Design review of the part built by this model. Coordinates are the model's own, in mm. Face numbers are marked on the shaded views. A direction names the side the tool comes from. Round coordinates to 2 decimals unless told otherwise and drop trailing zeros. Loops run counter-clockwise (first coordinate to the right, second up) from the corner with the lowest first, then second, coordinate; pieces in that order, holes last. Notation, with made-up numbers: (-13, 84.25) - (2, 84.25) arc R13 ccw to (2, 96.25) - close; hole circle Ø6 at (77, 14.5). An arc over 180 degrees is marked (long way). Use one line per item in the form item = value. Start each with the question number.
(1) Machinability: for the marked faces 1 and 2, which of the approach directions +Z, -Z, +X, -X, +Y, -Y give a long, thin tool a straight path to every point of the face, cutting with its end or side? Answer none if there is none.
(2) We need section D-D, the plane y = -17. Write out the cut boundary in (x, z).
(3) Wall thickness on probe 1 along Z at (x, y) = (-7, -2); probe 2 along Z at (x, y) = (-7.5, -3.45); probe 3 along Y at (x, z) = (-6, 7): over which ranges is each line inside the solid? List them lowest first. Write a range as [from, to].
(4) We need section A-A, the plane x = -15. Write out the cut boundary in (y, z).
(5) For pin 1 (1.9 mm diameter, centred on x = -7.5, z = 12.99, fed in from -Y); pin 2 (3 mm diameter, centred on x = -10.5, z = 15, fed in from -Y); pin 3 (4 mm diameter, centred on x = -1, y = -33.5, fed in from +Z); pin 4 (12 mm diameter, centred on x = -8.5, y = -10.5, fed in from +Z), all flat-tipped, find the tip position at first contact; note any pin that passes through.
(6) We need section C-C, the plane z = -4. Write out the cut boundary in (x, y), then the cut area to 3 significant figures.
(7) We need section B-B, the plane x = 7.5. Write out the cut boundary in (y, z), then the cut area to 3 significant figures.
from build123d import *

# Parameters (mm, degrees)
F0_R     = 21
F0_R_2   = 2
F0_R_3   = 5
F1_DEPTH = 6
F2_DEPTH = 38
F3_D     = 3.2


with BuildPart() as f1:
    # F0 (on Front) → F1 (new body)
    with BuildSketch(Plane.XZ):
        Circle(F0_R)
        with Locations((-7.5, -12.9903810568)):
            Circle(F0_R_2, mode=Mode.SUBTRACT)
        with Locations((7.5, -12.9903810568)):
            Circle(F0_R_2, mode=Mode.SUBTRACT)
        with Locations((-15, 0)):
            Circle(F0_R_2, mode=Mode.SUBTRACT)
        with Locations((-7.5, 12.9903810568)):
            Circle(F0_R_2, mode=Mode.SUBTRACT)
        Circle(F0_R_3, mode=Mode.SUBTRACT)
        with Locations((15, 0)):
            Circle(F0_R_2, mode=Mode.SUBTRACT)
        with Locations((7.5, 12.9903810568)):
            Circle(F0_R_2, mode=Mode.SUBTRACT)
        with Locations((-15, 0)):
            Circle(F0_R_2)
        with Locations((-7.5, 12.9903810568)):
            Circle(F0_R_2)
        with Locations((7.5, 12.9903810568)):
            Circle(F0_R_2)
        with Locations((15, 0)):
            Circle(F0_R_2)
        with Locations((7.5, -12.9903810568)):
            Circle(F0_R_2)
        with Locations((-7.5, -12.9903810568)):
            Circle(F0_R_2)
    extrude(amount=F1_DEPTH)

    # F0 (on Front) → F2 (join)
    with BuildSketch(Plane.XZ):
        Circle(F0_R_3)
        Circle(F0_R_2, mode=Mode.SUBTRACT)
        Circle(F0_R_2)
    extrude(amount=F2_DEPTH)

    # F3 (through all)
    with Locations(Plane(origin=(0, 0, 0), x_dir=(1, 0, 0), z_dir=(0, 1, 0))):
        with Locations((-15, 0), (-7.5, -12.9903810568), (7.5, -12.9903810568), (15, 0), (7.5, 12.9903810568), (-7.5, 12.9903810568), (0, 0)):
            Hole(F3_D / 2)


solid = f1.part
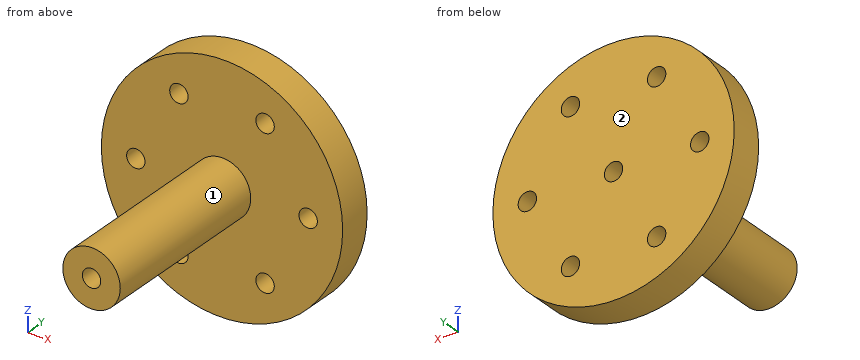
Data:
q1.face_1 = -Y
q1.face_2 = +Z, -Z, +X, -X, +Y
q2.outline = circle Ø10 at (0, 0); hole circle Ø3.2 at (0, 0)
q3.probe_1 = [-19.8, -14.51], [-11.47, 11.47], [14.51, 19.8]
q3.probe_2 = [-19.62, -14.59], [-11.39, 11.39], [14.59, 19.62]
q3.probe_3 = [-6, 0]
q4.outline = (-6, -14.7) - (0, -14.7) - (0, -1.6) - (-6, -1.6) - close; (-6, 1.6) - (0, 1.6) - (0, 14.7) - (-6, 14.7) - close
q5.pin_1 = through
q5.pin_2 = -6
q5.pin_3 = 5
q5.pin_4 = 20.51
q6.outline = (-20.62, -6) - (-3, -6) - (-3, -38) - (3, -38) - (3, -6) - (20.62, -6) - (20.62, 0) - (-20.62, 0) - close
q6.area = 439 mm^2
q7.outline = (-6, -19.62) - (0, -19.62) - (0, -14.59) - (-6, -14.59) - close; (-6, -11.39) - (0, -11.39) - (0, 11.39) - (-6, 11.39) - close; (-6, 14.59) - (0, 14.59) - (0, 19.62) - (-6, 19.62) - close
q7.area = 197 mm^2
